Autodesk Inventor part; units mm, degrees
ref_plane "YZ Plane" through (0, 0, 0) normal (1, 0, 0) x (0, 1, 0)
ref_plane "XZ Plane" through (0, 0, 0) normal (0, 1, 0) x (-1, 0, 0)
ref_plane "XY Plane" through (0, 0, 0) normal (0, 0, 1) x (1, 0, 0)
sketch "Sketch1" plane through (0, 0, 0) normal (0, 0, 1) x (1, 0, 0)
  line L0 (0, 0) -> (0, 8.6646) construction
  line L1 (20.9931, 1.27) -> (20.9931, 5.715)
  line L2 (20.9931, 5.715) -> (27.9781, 3.81)
  line L3 (27.9781, 3.81) -> (27.9781, 0)
  line L4 (27.9781, 0) -> (20.9931, 0)
  line L5 (20.9931, 1.27) -> (18.4531, 1.27)
  line L6 (18.4531, 1.27) -> (18.4531, 0)
  line L7 (18.4531, 0) -> (20.9931, 0)
  dimension "d0" = 20.9931
  dimension "d1" = 4.445
  dimension "d2" = 1.27
  dimension "d3" = 2.54
  dimension "d4" = 3.81
  dimension "d5" = 6.985
revolve "Revolution1" add sketch "Sketch1" angle 360 about axis through (0, 0, 0) along (0, 1, 0)
properties part number "Team Pin Base"
Here's how the part is built. I have some questions about the finished solid (model axes, mm). A direction names the side the tool comes from. Give positions to 0.01 mm unless a question says otherwise; leave off trailing zeros. Loops run counter-clockwise (first coordinate to the right, second up) from the corner with the lowest first, then second, coordinate; pieces in that order, holes last. Notation, with made-up numbers: M 59.25,-25.75 L 113.25,-25.75 A13 cw 113.25,-4.75 Z; hole C -1.75,-28 d9. An arc over 180 degrees is marked long. Use one line per item in the form item = value. Start each with the question number.
Q1. If we section it at A-A (x = 0): Write out the boundary of the cut face in (y, z) (3 decimals).
Q2. If we section it at B-B (y = 3): Write out the boundary of the cut face in (x, z).
Q3. I need wall thicknesses on line 1 along X through (y, z) = (0.85, 0); line 2 along X through (y, z) = (2.4, 0). Which ranges of each line are inside material? Lowest first, please.
Q4. Thinking about a two-plate mould opening in Z: for faces 3 (the flat face through (6, 0, 18)), 4 (the flat face through (0, 1.27, 19)), 5 (the cylindrical face through (26.686, 1.878, 8.404)), which applies, +Z half, -Z half, draft (parallel to the pull), parting line (faces both ways), or undercut?
Q5. Will these pins go through, and if not, where does the flat tip stop? pin 1 Ø1.5 at (y, z) = (3, 11) entering from +X; pin 2 Ø3 at (x, y) = (-12, 2) entering from +Z; pin 3 Ø3 at (x, y) = (-14, 1) entering from -Z.
Q6. Which directions (+Z, -Z, +X, -X, +Y, -Y) give clear straight access to the entire face, cutting with the end or side of a thin tool? Please do faces 1 (the cylindrical face through (-4, 0.626, -18.014)), 2 (the cylindrical face through (20.024, 3.524, -6.306)).
Taken from the geometry:
q1.outline = M 0,-27.978 L 3.81,-27.978 L 5.715,-20.993 L 1.27,-20.993 L 1.27,-18.453 L 0,-18.453 Z; M 0,18.453 L 1.27,18.453 L 1.27,20.993 L 5.715,20.993 L 3.81,27.978 L 0,27.978 Z
q2.outline = C 0,0 d55.96; hole C 0,0 d41.99
q3.line_1 = -27.98 to -18.45, 18.45 to 27.98
q3.line_2 = -27.98 to -20.99, 20.99 to 27.98
q4.face_3 = draft
q4.face_4 = undercut
q4.face_5 = parting line
q5.pin_1 = 26.03
q5.pin_2 = 25.93
q5.pin_3 = -25.03
q6.face_1 = +Y, -Y
q6.face_2 = +Y
